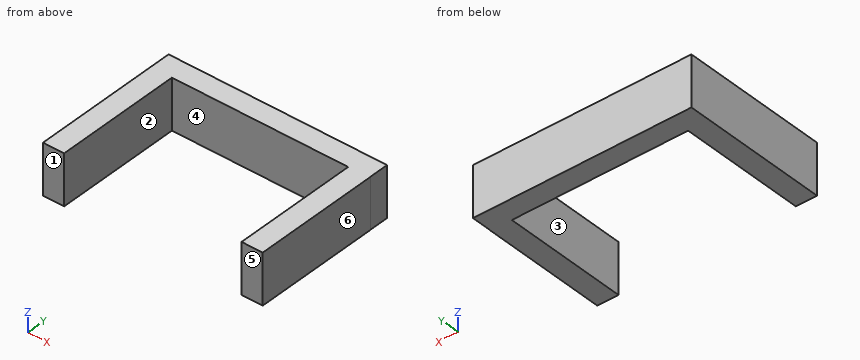
from build123d import *

# Parameters (mm, degrees)
F0_W     = 2.5180902779
F0_H     = 15.1024697029
F0_W_2   = 2.5
F0_H_2   = 0.1614799052
F1_DEPTH = 6


with BuildPart() as f1:
    # F0 (on Top) → F1 (new body)
    with BuildSketch(Plane.XY):
        Polygon((13, -0.3975302971), (13, 1.9409897977), (-13, 1.9409897977), (-13, -0.5590102023), (-10.4819097221, -0.5590102023), (10.5, -0.5590102023), (10.5, -0.3975302971), align=None)
        with Locations((-11.740954861, -8.1102450538)):
            Rectangle(F0_W, F0_H)
        Polygon((13.0180902779, -0.3975302971), (13, -0.3975302971), (13, -0.5590102023), (10.5, -0.5590102023), (10.5, -15.5), (13.0180902779, -15.5), align=None)
        with Locations((11.75, -0.4782702497)):
            Rectangle(F0_W_2, F0_H_2)
    extrude(amount=F1_DEPTH)


solid = f1.part
Here's how the part is built. I have some questions about the finished solid (model axes, mm). Face numbers are marked on the shaded views. A direction names the side the tool comes from. Round coordinates to 2 decimals unless told otherwise and drop trailing zeros. Order: outer loops, then holes, each group sorted by start corner. A loop starts at its lowest first (then second) coordinate and runs counter-clockwise, first axis right, second up. Notation, with made-up numbers: (59, 67.25) -> (97, 67.25) arc R21 ccw to (97, 96.25) -> close; hole circle Ø10 at (83.25, 44). An arc over 180 degrees is marked (long way). Return JSON: item names as keys, results as strings.
Q1. Which directions (+Z, -Z, +X, -X, +Y, -Y) give clear straight access to the entire face, cutting with the end or side of a thin tool? Please do the marked faces 1 and 2.
Filled sheet:
{"face 1": "+Z, -Z, +X, -X, -Y", "face 2": "+Z, -Z, -Y"}
Q2. For pin 1 Ø0.7 at (y, z) = (0.5, 4) entering from +X; pin 2 Ø3 at (x, z) = (12.5, 3) entering from -Y; pin 3 Ø8 at (x, y) = (-2.5, -11) entering from +Z; pin 4 Ø3 at (x, z) = (-1, 3) entering from -Y, each with a flat end and sliding along its axis, tell me the tip position at first contact or that it passes through.
Filled sheet:
{"pin 1": "stops at x = 13", "pin 2": "stops at y = -15.5", "pin 3": "passes through", "pin 4": "stops at y = -0.56"}
Q3. If we section it at C-C on x = 7.75: List the corners of the cut face in (y, z) for me.
Filled sheet:
{"outline": "(-0.56, 0) -> (1.94, 0) -> (1.94, 6) -> (-0.56, 6) -> close"}
Q4. If we section it at A-A on y = -5.75: List the corners of the cut face in (x, z) for me, plus the area to 3 significant figures.
Filled sheet:
{"outline": "(-13, 0) -> (-10.48, 0) -> (-10.48, 6) -> (-13, 6) -> close; (10.5, 0) -> (13.02, 0) -> (13.02, 6) -> (10.5, 6) -> close", "area": "30.2 mm^2"}
Q5. I need wall thicknesses on line 1 along X through (y, z) = (-14.5, 4.65); line 2 along Y through (x, z) = (-9.5, 1.3); line 3 along X through (y, z) = (-0.25, 4.4). Which ranges of each line are inside material? Lowest first, please. Write a range as from..to.
Filled sheet:
{"line 1": "x = -13..-10.48, 10.5..13.02", "line 2": "y = -0.56..1.94", "line 3": "x = -13..13"}
Q6. If we mould it in two halves opening along X, with no side actions, what happens to the marked faces 3, 4, 5 and 6? For each: released by +X, released by -X, zero draft, split by the parting line, or undercut.
Filled sheet:
{"face 3": "undercut", "face 4": "undercut", "face 5": "zero draft", "face 6": "released by +X"}
